from build123d import *

# Parameters (mm, degrees)
ESQUISSE1_W             = 71.1
ESQUISSE1_H             = 24.3
BOSS_EXTRU_1_DEPTH      = 7
CONG_1_R                = 0.5
ESQUISSE2_W             = 1.653567917
ESQUISSE2_H             = 1.375254205
ESQUISSE2_W_2           = 1.332598991
ESQUISSE2_H_2           = 1.640495544
ESQUISSE2_W_3           = 1.790407611
ESQUISSE2_H_3           = 2.285395674
ENL_V_MAT_EXTRU_1_DEPTH = 7
ESQUISSE3_W             = 64.4
ESQUISSE3_H             = 14.5
ENL_V_MAT_EXTRU_2_DEPTH = 0.7
ESQUISSE4_W             = 7
ESQUISSE4_H             = 0.5
BOSS_EXTRU_2_DEPTH      = 1.6
BOSS_EXTRU_3_DEPTH      = 2.2


with BuildPart() as part:
    # Esquisse1 → Boss.-Extru.1 (new body)
    with BuildSketch(Plane(origin=(0, 0, 0), x_dir=(1, 0, 0), z_dir=(0, 1, 0))):
        with Locations((35.55, 12.15)):
            Rectangle(ESQUISSE1_W, ESQUISSE1_H)
    extrude(amount=BOSS_EXTRU_1_DEPTH)

    # Congé1
    cong_1_edges = [part.edges().sort_by_distance(p)[0] for p in [
        (71.1, 7, -12.15),
        (35.55, 7, -24.3),
        (0, 7, -12.15),
        (35.55, 7, 0),
    ]]
    fillet(cong_1_edges, radius=CONG_1_R)

    # Esquisse2 → Enlèv. mat.-Extru.1 (cut)
    with BuildSketch(Plane(origin=(0, 7, 0), x_dir=(1, 0, 0), z_dir=(0, 1, 0))):
        with Locations((-0.326783959, 24.487627102)):
            Rectangle(ESQUISSE2_W, ESQUISSE2_H)
        with Locations((-0.166299496, -0.320247772)):
            Rectangle(ESQUISSE2_W_2, ESQUISSE2_H_2)
        with Locations((71.495203806, -0.320247772)):
            Rectangle(ESQUISSE2_W_3, ESQUISSE2_H_2)
        with Locations((71.495203806, 24.942697837)):
            Rectangle(ESQUISSE2_W_3, ESQUISSE2_H_3)
    extrude(amount=-ENL_V_MAT_EXTRU_1_DEPTH, mode=Mode.SUBTRACT)

    # Esquisse3 → Enlèv. mat.-Extru.2 (cut)
    with BuildSketch(Plane(origin=(0, 7, 0), x_dir=(1, 0, 0), z_dir=(0, 1, 0))):
        with Locations((35.55, 12.15)):
            Rectangle(ESQUISSE3_W, ESQUISSE3_H)
    extrude(amount=-ENL_V_MAT_EXTRU_2_DEPTH, mode=Mode.SUBTRACT)

    # Esquisse4 → Boss.-Extru.2 (add)
    with BuildSketch(Plane(origin=(0, 0, 0), x_dir=(-1, 0, 0), z_dir=(0, -1, 0))):
        with Locations((-6.5, 0.25)):
            Rectangle(ESQUISSE4_W, ESQUISSE4_H)
        with Locations((-6.5, 24.05)):
            Rectangle(ESQUISSE4_W, ESQUISSE4_H)
        with Locations((-35.55, 0.25)):
            Rectangle(ESQUISSE4_W, ESQUISSE4_H)
        with Locations((-35.55, 24.05)):
            Rectangle(ESQUISSE4_W, ESQUISSE4_H)
        with Locations((-64.6, 0.25)):
            Rectangle(ESQUISSE4_W, ESQUISSE4_H)
        with Locations((-64.6, 24.05)):
            Rectangle(ESQUISSE4_W, ESQUISSE4_H)
    extrude(amount=BOSS_EXTRU_2_DEPTH)

    # Esquisse5 → Boss.-Extru.3 (add)
    with BuildSketch(Plane.XZ.offset(1.6)):
        Polygon((4.385314947, -3.562636494), (4.731995615, -3.8), (6.991422348, -0.5), (10, -0.5), (10, 0), (6.824562261, 0), align=None)
        Polygon((33.435314947, -3.562636494), (33.781995615, -3.8), (36.041422348, -0.5), (39.05, -0.5), (39.05, 0), (35.874562261, 0), align=None)
        Polygon((65.091422348, -0.5), (64.582224877, -0.5), (62.485314947, -3.562636494), (62.831995615, -3.8), align=None)
        Polygon((68.1, -0.5), (68.1, 0), (64.924562261, 0), (64.582224877, -0.5), (65.091422348, -0.5), align=None)
        Polygon((66.714685053, -20.737363506), (66.368004385, -20.5), (64.108577652, -23.8), (61.1, -23.8), (61.1, -24.3), (64.275437739, -24.3), align=None)
        Polygon((8.614685053, -20.737363506), (8.268004385, -20.5), (6.008577652, -23.8), (3, -23.8), (3, -24.3), (6.175437739, -24.3), align=None)
        Polygon((37.664685053, -20.737363506), (37.318004385, -20.5), (35.058577652, -23.8), (32.05, -23.8), (32.05, -24.3), (35.225437739, -24.3), align=None)
    extrude(amount=BOSS_EXTRU_3_DEPTH)


solid = part.part
The listing builds one solid part. Answer for the finished solid, in the listing's coordinates (mm). A direction names the side the tool comes from. Coordinates: 2 decimals unless noted, no trailing zeros. Write each loop counter-clockwise with the first axis right and the second up, starting at its lowest first coordinate (ties: lowest second). Pieces come first, ordered by that corner, then holes. Notation, with made-up numbers: (83, 18.25) -> (90, 18.25) arc R22 cw to (90, 34.25) -> close; hole circle Ø7 at (30.25, -36.5). An arc over 180 degrees is marked (long way). One line per question, with ' | ' between items.
1. Straight lines are drawn through the part: line 1 (Z direction, x = 39, y = 6.5); line 2 (Y direction, x = 16.5, z = -1); line 3 (Y direction, x = 13, z = -17.75). For each, find the intervals that lie inside material, in ascending order.
Verdict:
line 1: z = -24.3 to -19.4, -4.9 to 0 | line 2: y = 0 to 7 | line 3: y = 0 to 6.3
2. For a pull along Y with two mould halves and no side action, classify faces 5 (the flat face through (35, 7, -20)), 6 (the flat face through (35, 2, -24.3)), 7 (the flat face through (35.6, -3.8, -0.8)), 8 (the flat face through (7.3, -1.6, -22.3)) as released by +Y, released by -Y, zero draft, split by the parting line, or undercut.
Verdict:
face 5: released by +Y | face 6: zero draft | face 7: released by -Y | face 8: undercut
3. Section B-B (z = -22) is taken. Determine the outline of the cut face in (x, y), and give its area (3 significant figures).
Verdict:
outline: (0, 0) -> (71.1, 0) -> (71.1, 6.5) arc R0.5 ccw to (70.6, 7) -> (0.5, 7) arc R0.5 ccw to (0, 6.5) -> close; (7.24, -3.8) -> (7.75, -3.8) -> (7.75, -1.6) -> (7.24, -1.6) -> close; (36.29, -3.8) -> (36.8, -3.8) -> (36.8, -1.6) -> (36.29, -1.6) -> close; (65.34, -3.8) -> (65.85, -3.8) -> (65.85, -1.6) -> (65.34, -1.6) -> close | area: 501 mm^2
4. Section C-C (z = -8) is taken. Determine the outline of the cut face in (x, y).
Verdict:
outline: (0, 0) -> (71.1, 0) -> (71.1, 6.5) arc R0.5 ccw to (70.6, 7) -> (67.75, 7) -> (67.75, 6.3) -> (3.35, 6.3) -> (3.35, 7) -> (0.5, 7) arc R0.5 ccw to (0, 6.5) -> close
5. Section A-A (x = 20.5) is taken. Determine the outline of the cut face in (y, z), and give its area (3 significant figures).
Verdict:
outline: (0, -24.3) -> (6.5, -24.3) arc R0.5 ccw to (7, -23.8) -> (7, -19.4) -> (6.3, -19.4) -> (6.3, -4.9) -> (7, -4.9) -> (7, -0.5) arc R0.5 ccw to (6.5, 0) -> (0, 0) -> close | area: 160 mm^2
6. Given pin 1 Ø0.6 at (y, z) = (-1, -24) entering from +X; pin 2 Ø4.5 at (x, z) = (24.5, -10.5) entering from +Y; pin 3 Ø6 at (x, z) = (33, -14.5) entering from -Y, each flat-ended and moving along its own axis, determine where each tip first touches the part or whether it passes through.
Verdict:
pin 1: stops at x = 68.1 | pin 2: stops at y = 6.3 | pin 3: stops at y = 0
7. Which of the six approach directions +Z, -Z, +X, -X, +Y, -Y give full straight-line access (tool end or side, diameter ignored) to faces 1 (the flat face through (7.15, -2.68, -22.13)), 2 (the flat face through (35, 6.3, -12)), 3 (the flat face through (65.48, -2.68, -22.54)), 4 (the flat face through (5.62, -2.68, -1.76))?
Verdict:
face 1: -X, -Y | face 2: +Y | face 3: -Z, +X, -Y | face 4: +Z, -X, -Y
